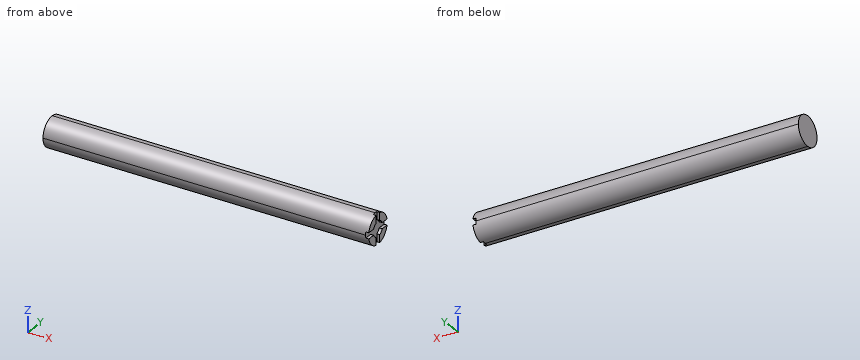
```python
from build123d import *

# Parameters (mm, degrees)
F0_W        = 25.4
F0_H        = 25.4
F1_DEPTH    = 279.4
F3_DEPTH    = 2.54
F4_T1_DEPTH = 342.9


# Not quite as in the source:
# - a fillet or chamfer that OpenCascade refuses, or shapes differently, is made with other operations: its cross-section is extruded or revolved along the edge and cut away or added


with BuildPart() as f1:
    # F0 (on Right) → F1 (new body)
    with BuildSketch(Plane.YZ):
        with Locations((12.7, 12.7)):
            Rectangle(F0_W, F0_H)
    extrude(amount=F1_DEPTH)

    # F2 (on face) → F3 (cut)
    with BuildSketch(Plane.YZ.offset(279.4)):
        with BuildLine():
            Line((15.24, 25.4), (12.7, 25.4))
            Line((12.7, 25.4), (12.7, 19.05))
            ThreePointArc((12.7, 19.05), (13.9973662374, 18.9160550871), (15.24, 18.5198711326))
            Line((15.24, 18.5198711326), (15.24, 25.4))
        make_face()
        with BuildLine():
            Line((12.7, 19.05), (12.7, 25.4))
            Line((12.7, 25.4), (10.16, 25.4))
            Line((10.16, 25.4), (10.16, 18.5198711326))
            ThreePointArc((10.16, 18.5198711326), (11.4026337626, 18.9160550871), (12.7, 19.05))
        make_face()
        with BuildLine():
            ThreePointArc((15.24, 18.5198711326), (13.9973662374, 18.9160550871), (12.7, 19.05))
            Line((12.7, 19.05), (12.7, 18.5198711326))
            Line((12.7, 18.5198711326), (15.24, 18.5198711326))
        make_face()
        with BuildLine():
            Line((12.7, 18.5198711326), (12.7, 19.05))
            ThreePointArc((12.7, 19.05), (11.4026337626, 18.9160550871), (10.16, 18.5198711326))
            Line((10.16, 18.5198711326), (12.7, 18.5198711326))
        make_face()
        with BuildLine():
            Line((15.24, 18.5198711326), (12.7, 18.5198711326))
            Line((12.7, 18.5198711326), (10.16, 18.5198711326))
            ThreePointArc((10.16, 18.5198711326), (8.2098719395, 17.1901280605), (6.8801288674, 15.24))
            ThreePointArc((6.8801288674, 15.24), (6.35, 12.7), (6.8801288674, 10.16))
            ThreePointArc((6.8801288674, 10.16), (8.2098719395, 8.2098719395), (10.16, 6.8801288674))
            Line((10.16, 6.8801288674), (15.24, 6.8801288674))
            ThreePointArc((15.24, 6.8801288674), (17.1901280605, 8.2098719395), (18.5198711326, 10.16))
            ThreePointArc((18.5198711326, 10.16), (18.9160550871, 11.4026337626), (19.05, 12.7))
            ThreePointArc((19.05, 12.7), (18.9160550871, 13.9973662374), (18.5198711326, 15.24))
            ThreePointArc((18.5198711326, 15.24), (17.1901280605, 17.1901280605), (15.24, 18.5198711326))
        make_face()
        with BuildLine():
            Line((25.4, 15.24), (18.5198711326, 15.24))
            ThreePointArc((18.5198711326, 15.24), (18.9160550871, 13.9973662374), (19.05, 12.7))
            ThreePointArc((19.05, 12.7), (18.9160550871, 11.4026337626), (18.5198711326, 10.16))
            Line((18.5198711326, 10.16), (25.4, 10.16))
            Line((25.4, 10.16), (25.4, 15.24))
        make_face()
        with BuildLine():
            ThreePointArc((6.8801288674, 10.16), (6.35, 12.7), (6.8801288674, 15.24))
            Line((6.8801288674, 15.24), (0, 15.24))
            Line((0, 15.24), (0, 10.16))
            Line((0, 10.16), (6.8801288674, 10.16))
        make_face()
        with BuildLine():
            Line((15.24, 6.8801288674), (10.16, 6.8801288674))
            ThreePointArc((10.16, 6.8801288674), (12.7, 6.35), (15.24, 6.8801288674))
        make_face()
        with BuildLine():
            ThreePointArc((15.24, 6.8801288674), (12.7, 6.35), (10.16, 6.8801288674))
            Line((10.16, 6.8801288674), (10.16, 0))
            Line((10.16, 0), (15.24, 0))
            Line((15.24, 0), (15.24, 6.8801288674))
        make_face()
    extrude(amount=-F3_DEPTH, mode=Mode.SUBTRACT)

    # F4: fillet of radius 12.7 on 4 edges, made by hand

    # F4_s2 → F4_t1 (cut)
    with BuildSketch(Plane.YZ.offset(-31.75)):
        with BuildLine():
            ThreePointArc((12.7, 25.4), (21.6802561211, 21.6802561211), (25.4, 12.7))
            Line((25.4, 12.7), (25.4, 25.4))
            Line((25.4, 25.4), (12.7, 25.4))
        make_face()
        with BuildLine():
            ThreePointArc((12.7, 0), (21.6802561211, 3.7197438789), (25.4, 12.7))
            Line((25.4, 12.7), (25.4, 0))
            Line((25.4, 0), (12.7, 0))
        make_face()
        with BuildLine():
            ThreePointArc((0, 12.7), (3.7197438789, 21.6802561211), (12.7, 25.4))
            Line((12.7, 25.4), (0, 25.4))
            Line((0, 25.4), (0, 12.7))
        make_face()
        with BuildLine():
            ThreePointArc((0, 12.7), (3.7197438789, 3.7197438789), (12.7, 0))
            Line((12.7, 0), (0, 0))
            Line((0, 0), (0, 12.7))
        make_face()
    extrude(amount=F4_T1_DEPTH, mode=Mode.SUBTRACT)


solid = f1.part
```
Design review of the part built by this model. Coordinates are the model's own, in mm. Give positions to 0.01 mm unless a question says otherwise; leave off trailing zeros. Loops run counter-clockwise (first coordinate to the right, second up) from the corner with the lowest first, then second, coordinate; pieces in that order, holes last. Notation, with made-up numbers: M 22.25,12 L 29.25,12 A34 cw 29.25,49 Z; hole C -17,61.25 d2. An arc over 180 degrees is marked long. Return JSON: item names as keys, results as strings. Group by question number.
Item 1: Insertion check: pin 1 Ø1.3 at (x, y) = (278.5, 22.5) entering from +Z; pin 2 Ø3 at (x, z) = (278, 2.5) entering from -Y; pin 3 Ø2 at (x, z) = (278, 5) entering from +Y. Each pin has a flat end and moves straight along its axis. Give the tip position at first contact, or say it passes through.
Item 2: For probe 1 along Y at (x, z) = (143.5, 13); probe 2 along X at (y, z) = (15.5, 15), list the stretches that pass through material, from the lowest coordinate up.
Item 3: We need section B-B (x = 62.5). Give the boundary of the cut face in (y, z), and give its area (3 significant figures).
Item 4: We need section A-A (z = 21.5). Give the boundary of the cut face in (x, y).
Output:
{
 "1": {"pin 1": "stops at z = 21.51", "pin 2": "stops at y = 3.45", "pin 3": "stops at y = 23.49"},
 "2": {"probe 1": "y = 0 to 25.4", "probe 2": "x = 0 to 276.86"},
 "3": {"outline": "C 12.7,12.7 d25.4", "area": "507 mm^2"},
 "4": {"outline": "M 0,3.54 L 279.4,3.54 L 279.4,10.16 L 276.86,10.16 L 276.86,15.24 L 279.4,15.24 L 279.4,21.86 L 0,21.86 Z"}
}
